```python
from build123d import *

# Parameters (mm, degrees)
F0_R     = 10
F1_DEPTH = 1.5
F2_R     = 3.95
F2_R_2   = 2.25
F3_DEPTH = 7.1
F4_SIZE  = 0.5


with BuildPart() as f1:
    # F0 (on Top) → F1 (new body)
    with BuildSketch(Plane.XY):
        Circle(F0_R)
    extrude(amount=F1_DEPTH)

    # F2 (on face) → F3 (join)
    with BuildSketch(Plane.XY.offset(1.5)):
        Circle(F2_R)
        Circle(F2_R_2, mode=Mode.SUBTRACT)
    extrude(amount=F3_DEPTH)

    # F4
    f4_edges = [f1.edges().sort_by_distance(p)[0] for p in [
        (-3.95, 0, 8.6),
        (-2.25, 0, 8.6),
    ]]
    chamfer(f4_edges, length=F4_SIZE)


solid = f1.part
```
Work out the finished part from the listing and answer in its coordinate system (mm). A direction names the side the tool comes from. Round coordinates to 2 decimals unless told otherwise and drop trailing zeros. Loops run counter-clockwise (first coordinate to the right, second up) from the corner with the lowest first, then second, coordinate; pieces in that order, holes last.
(1) For faces 4 (the cylindrical face through (-3.135, -2.404, 4.754)), 5 (the flat face through (0, 0, 0)), determine the directions among +Z, -Z, +X, -X, +Y, -Y from which every point of the face is accessible in a straight line to the end or side of a thin tool.
Computed values:
face 4: +Z
face 5: -Z, +X, -X, +Y, -Y
(2) The part is cut by section C-C, the plane z = 5. Give the vertices of the cut face in (x, y).
Computed values:
outline: circle Ø7.9 at (0, 0); hole circle Ø4.5 at (0, 0)
(3) The mould has two halves that part along X. Classify faces 1 (the cylindrical face through (-2.17, -9.76, 0.74)), 2 (the cylindrical face through (-0.29, 2.23, 4.75)), 3 (the flat face through (-3, -1, 8.6)): pulls with the +X half, pulls with the -X half, needs draft (parallel to the pull), parting line crosses it, or undercut.
Computed values:
face 1: parting line crosses it
face 2: undercut
face 3: needs draft
(4) Find the intervals of material crossed by L1, parallel to Y at x = 0, z = 3; L2, parallel to Z at x = 8.75, y = 4.5; L3, parallel to Y at x = 1.5, z = 5, in increasing order.
Computed values:
L1: y = -3.95 to -2.25, 2.25 to 3.95
L2: z = 0 to 1.5
L3: y = -3.65 to -1.68, 1.68 to 3.65
(5) Each of these flat-tipped pins is pushed along its axis until it touches: P1, Ø5, axis at x = -6, z = 5.5, coming from the +Y side; P2, Ø3, axis at x = -5, z = 1.5, coming from the +Y side; P3, Ø1.5, axis at y = 0, z = 5.5, coming from the +X side. Where does it stop, or does it pass through?
Computed values:
P1: stops at y = 1.83
P2: stops at y = 9.37
P3: stops at x = 3.95
(6) The part is cut by section D-D, the plane z = 1. Give the vertices of the cut face in (x, y).
Computed values:
outline: circle Ø20 at (0, 0)
(7) The part is cut by section A-A, the plane y = 0. Give the vertices of the cut face in (x, z).
Computed values:
outline: (-10, 0) - (10, 0) - (10, 1.5) - (3.95, 1.5) - (3.95, 8.1) - (3.45, 8.6) - (2.75, 8.6) - (2.25, 8.1) - (2.25, 1.5) - (-2.25, 1.5) - (-2.25, 8.1) - (-2.75, 8.6) - (-3.45, 8.6) - (-3.95, 8.1) - (-3.95, 1.5) - (-10, 1.5) - close
